from build123d import *

# Parameters (mm, degrees)
SKETCH1_W               = 24
SKETCH1_H               = 53
BOSS_EXTRUDE1_DEPTH     = 2
BOSS_EXTRUDE2_DEPTH     = 53
SKETCH3_W               = 10.2
SKETCH3_H               = 49.4
CUT_EXTRUDE1_DEPTH      = 9.6
CUT_EXTRUDE2_DEPTH      = 32.317886263
CUT_EXTRUDE2_DEPTH_BACK = 32.317886263


with BuildPart() as part:
    # Sketch1 → Boss-Extrude1 (new body)
    with BuildSketch(Plane.XY):
        Rectangle(SKETCH1_W, SKETCH1_H)
    extrude(amount=BOSS_EXTRUDE1_DEPTH)

    # Sketch2 → Boss-Extrude2 (add)
    with BuildSketch(Plane.XZ.offset(26.5)):
        with BuildLine():
            Line((-8.4, 11.6), (8.4, 11.6))
            ThreePointArc((8.4, 11.6), (10.945584412, 10.545584412), (12, 8))
            Line((12, 8), (12, 2))
            Line((12, 2), (-12, 2))
            Line((-12, 2), (-12, 8))
            ThreePointArc((-12, 8), (-10.945584412, 10.545584412), (-8.4, 11.6))
        make_face()
    extrude(amount=-BOSS_EXTRUDE2_DEPTH)

    # Sketch3 → Cut-Extrude1 (cut)
    with BuildSketch(Plane.XY.offset(11.6)):
        with Locations((5.6, 0)):
            Rectangle(SKETCH3_W, SKETCH3_H)
        with Locations((-5.6, 0)):
            Rectangle(SKETCH3_W, SKETCH3_H)
    extrude(amount=-CUT_EXTRUDE1_DEPTH, mode=Mode.SUBTRACT)

    # Sketch4 → Cut-Extrude2 (cut, two sides: drawn at the far end of the back side and taken through both)
    with BuildSketch(Plane(origin=(0, 0, 0), x_dir=(0, 0, -1), z_dir=(1, 0, 0)).offset(-CUT_EXTRUDE2_DEPTH_BACK)):
        Polygon((-16.6, -15.119912853), (-16.6, 15.119912853), (-6, 9), (-6, -9), align=None)
    extrude(amount=CUT_EXTRUDE2_DEPTH + CUT_EXTRUDE2_DEPTH_BACK, mode=Mode.SUBTRACT)


solid = part.part
Work out the finished part from the listing and answer in its coordinate system (mm). A direction names the side the tool comes from. Give positions to 0.01 mm unless a question says otherwise; leave off trailing zeros. Order: outer loops, then holes, each group sorted by start corner. A loop starts at its lowest first (then second) coordinate and runs counter-clockwise, first axis right, second up. Notation, with made-up numbers: (89.25, -31.5) - (144.25, -31.5) arc R29 ccw to (144.25, 1.5) - close; hole circle Ø2 at (35.25, 41). An arc over 180 degrees is marked (long way). Answer as CSV lines item,"result". Start each with the question number.
Q1. For faces 1 (the face through (-6, -24.7, 7)), 2 (the face through (-11.36, -10.05, 7.82)), 3 (the face through (-11.679, 20.029, 9.485)), determine the directions among +Z, -Z, +X, -X, +Y, -Y from which every point of the face is accessible in a straight line to the end or side of a thin tool.
Q2. The part is cut by section B-B (y = 7). Write down the section's boundary in (x, z), then the cut area to 3 significant figures.
Q3. The part is cut by section A-A (z = 2.5). Write down the section's boundary in (x, y).
Q4. Given pin 1 Ø1 at (x, y) = (-11, 4) entering from +Z; pin 2 Ø5 at (x, y) = (-3.5, -0.5) entering from +Z, each flat-ended and moving along its own axis, determine where each tip first touches the part or whether it passes through.
Q5. The mould has two halves that part along Y. Classify faces 4 (the face through (0, 26.5, 6)), 5 (the face through (0, -24, 11.6)), 6 (the face through (-6, 0, 2)): +Y half, -Y half, draft (parallel to the pull), parting line (faces both ways), or undercut.
Q6. Find the intervals of material crossed by L1, parallel to X at y = 5.5, z = 2.5; L2, parallel to Y at x = -3.75, z = 11; L3, parallel to Z at x = -10.5, y = 19.5, in increasing order. Write a range as [from, to].
Q7. The part is cut by section D-D (z = 10.25). Write down the section's boundary in (x, y).
Q8. The part is cut by section C-C (x = 3.5). Write down the section's boundary in (y, z), then the cut area to 3 significant figures.
Check result:
1,face 1,"+Z"
1,face 2,"+Z, +X, -X"
1,face 3,"+Z, -X, +Y, -Y"
2,outline,"(-12, 0) - (12, 0) - (12, 6) - (10.7, 6) - (10.7, 2) - (0.5, 2) - (0.5, 6) - (-0.5, 6) - (-0.5, 2) - (-10.7, 2) - (-10.7, 6) - (-12, 6) - close"
2,area,"62.4 mm²"
3,outline,"(-12, -26.5) - (12, -26.5) - (12, 26.5) - (-12, 26.5) - close; hole (-10.7, -24.7) - (-0.5, -24.7) - (-0.5, 24.7) - (-10.7, 24.7) - close; hole (0.5, -24.7) - (10.7, -24.7) - (10.7, 24.7) - (0.5, 24.7) - close"
4,pin 1,"stops at z = 6"
4,pin 2,"stops at z = 2"
5,face 4,"+Y half"
5,face 5,"draft"
5,face 6,"undercut"
6,L1,"x = [-12, -10.7], [-0.5, 0.5], [10.7, 12]"
6,L2,"y = [-26.5, -24.7], [24.7, 26.5]"
6,L3,"z = [0, 2]"
7,outline,"(-11.21, -26.5) - (11.21, -26.5) - (11.21, -11.45) - (10.7, -11.45) - (10.7, -24.7) - (0.5, -24.7) - (0.5, -11.45) - (-0.5, -11.45) - (-0.5, -24.7) - (-10.7, -24.7) - (-10.7, -11.45) - (-11.21, -11.45) - close; (-11.21, 11.45) - (-10.7, 11.45) - (-10.7, 24.7) - (-0.5, 24.7) - (-0.5, 11.45) - (0.5, 11.45) - (0.5, 24.7) - (10.7, 24.7) - (10.7, 11.45) - (11.21, 11.45) - (11.21, 26.5) - (-11.21, 26.5) - close"
8,outline,"(-26.5, 0) - (26.5, 0) - (26.5, 11.6) - (24.7, 11.6) - (24.7, 2) - (-24.7, 2) - (-24.7, 11.6) - (-26.5, 11.6) - close"
8,area,"141 mm²"
